```python
from build123d import *

# Parameters (mm, degrees)
SKETCH1_R           = 3
BOSS_EXTRUDE1_DEPTH = 6


with BuildPart() as part:
    # Sketch1 → Boss-Extrude1 (new body)
    with BuildSketch(Plane.XY):
        with BuildLine():
            Line((29.097558797, 17.5), (24.40844793, 25.621778265))
            ThreePointArc((24.40844793, 25.621778265), (24.40844793, 36.592231664), (35.378901329, 36.592231664))
            ThreePointArc((35.378901329, 36.592231664), (35.506003821, 36.393205072), (35.627115001, 36.190476904))
            Line((35.627115001, 36.190476904), (42.087939854, 25))
            ThreePointArc((42.087939854, 25), (48.786669665, 0), (42.087939854, -25))
            Line((42.087939854, -25), (35.389210043, -36.602540378))
            ThreePointArc((35.389210043, -36.602540378), (25.685911427, -35.325076881), (24.40844793, -25.621778265))
            Line((24.40844793, -25.621778265), (29.097558797, -17.5))
            ThreePointArc((29.097558797, -17.5), (33.786669665, 0), (29.097558797, 17.5))
        make_face()
        with Locations((41.286669665, 0)):
            Circle(SKETCH1_R, mode=Mode.SUBTRACT)
        with Locations((30.212002479, -31.425332814)):
            Circle(SKETCH1_R, mode=Mode.SUBTRACT)
        with Locations((29.893674629, 31.107004965)):
            Circle(SKETCH1_R, mode=Mode.SUBTRACT)
    extrude(amount=BOSS_EXTRUDE1_DEPTH)


solid = part.part
```
Source: CAD feature listing. Evaluate the final solid. Frame: model axes, mm. A direction names the side the tool comes from. Coordinates: 2 decimals unless noted, no trailing zeros. Loops run counter-clockwise (first coordinate to the right, second up) from the corner with the lowest first, then second, coordinate; pieces in that order, holes last. Notation, with made-up numbers: (61.5, 4) - (102.5, 4) arc R29 ccw to (102.5, 29) - close; hole circle Ø3 at (-34.75, 54). An arc over 180 degrees is marked (long way). Answer as CSV lines item,"result".
1. Ray query, line 1 (Y direction, x = 30, z = 2.35); line 2 (Y direction, x = 31.25, z = 5.5); line 3 (X direction, y = 1, z = 5.5). Return the intervals inside material, ascending.
Established:
line 1,"y = -37.56 to -34.42, -28.43 to -15.83, 15.83 to 28.11, 34.11 to 38.86"
line 2,"y = -37.68 to -34.24, -28.61 to -13.08, 13.08 to 28.43, 33.78 to 38.74"
line 3,"x = 33.77 to 38.46, 44.12 to 48.78"
2. Mould query, pull axis Y, two halves, no side actions, for faces 1 (the cylindrical face through (38.29, 0.13, 2.96)), 2 (the flat face through (36, 1, 6)), 3 (the flat face through (38.812, 30.674, 2.958)). Classes: released by +Y, released by -Y, zero draft, split by the parting line, or undercut.
Established:
face 1,"undercut"
face 2,"zero draft"
face 3,"released by +Y"
3. Section C-C (z = 1.65). Return loops of the section in (x, y).
Established:
outline,"(24.41, -25.62) arc R8.04 ccw to (35.39, -36.6) - (42.09, -25) arc R50 ccw to (42.09, 25) - (35.63, 36.19) arc R7.92 ccw to (35.38, 36.59) arc R7.76 ccw to (24.41, 25.62) - (29.1, 17.5) arc R35 cw to (29.1, -17.5) - close; hole circle Ø6 at (29.89, 31.11); hole circle Ø6 at (30.21, -31.43); hole circle Ø6 at (41.29, 0)"
4. Reachability of faces 4 (the flat face through (26.79, 21.5, 2.96)), 5 (the cylindrical face through (27.5, 29.3, 3)) from +Z, -Z, +X, -X, +Y, -Y: full face, straight path, thin tool, end or side. Return the list, or none.
Established:
face 4,"+Z, -Z, -X"
face 5,"+Z, -Z"
5. Section A-A (y = 0). Return loops of the section in (x, z).
Established:
outline,"(33.79, 0) - (38.29, 0) - (38.29, 6) - (33.79, 6) - close; (44.29, 0) - (48.79, 0) - (48.79, 6) - (44.29, 6) - close"
6. Contact query for flat-ended pins moving along their axis: pin 1 (2 mm diameter, centred on x = 35.5, y = 21.5, fed in from -Z); pin 2 (2 mm diameter, centred on x = 40, z = 1.5, fed in from +Y); pin 3 (5 mm diameter, centred on x = 30.21, y = -31.43, fed in from -Z). Output: stop coordinate, or through.
Established:
pin 1,"stops at z = 0"
pin 2,"stops at y = 30.35"
pin 3,"passes through"
7. Section B-B (x = 30). Return loops of the section in (y, z), then the cut area to 3 significant figures.
Established:
outline,"(-37.56, 0) - (-34.42, 0) - (-34.42, 6) - (-37.56, 6) - close; (-28.43, 0) - (-15.83, 0) - (-15.83, 6) - (-28.43, 6) - close; (15.83, 0) - (28.11, 0) - (28.11, 6) - (15.83, 6) - close; (34.11, 0) - (38.86, 0) - (38.86, 6) - (34.11, 6) - close"
area,"197 mm2"
8. Section D-D (y = 33). Return loops of the section in (x, z).
Established:
outline,"(22.37, 0) - (27.57, 0) - (27.57, 6) - (22.37, 6) - close; (32.22, 0) - (37.47, 0) - (37.47, 6) - (32.22, 6) - close"
